from build123d import *

# Parameters (mm, degrees)
PAD_DEPTH       = 15
SKETCH001_W     = 12
SKETCH001_H     = 5.5
POCKET_DEPTH    = 12.001
SKETCH002_R     = 2.25
POCKET001_DEPTH = 20.001
CHAMFER_SIZE    = 1.5
CHAMFER001_SIZE = 2.5
CHAMFER002_SIZE = 0.5


with BuildPart() as part:
    # Sketch → Pad (new body)
    with BuildSketch(Plane.XZ):
        Polygon((-6, 20), (-4.1, 20), (-4.1, 5), (4.1, 5), (4.1, 20), (6, 20), (6, 0), (-6, 0), align=None)
    extrude(amount=PAD_DEPTH)

    # Sketch001 (on Face2 of Pad) → Pocket (cut, through all)
    with BuildSketch(Plane(origin=(6, 0, 0), x_dir=(0, 0, 1), z_dir=(1, 0, 0))):
        with Locations((13, 7.5)):
            Rectangle(SKETCH001_W, SKETCH001_H)
    extrude(amount=-POCKET_DEPTH, mode=Mode.SUBTRACT)

    # Sketch002 (on Face11 of Pocket) → Pocket001 (cut, through all)
    with BuildSketch(Plane(origin=(0, 0, 0), x_dir=(1, 0, 0), z_dir=(0, 0, -1))):
        with Locations((0, 7.5)):
            Circle(SKETCH002_R)
    extrude(amount=-POCKET001_DEPTH, mode=Mode.SUBTRACT)

    # Chamfer
    chamfer_edges = [part.edges().sort_by_distance(p)[0] for p in [
        (6, -4.75, 13),
        (6, -10.25, 13),
        (-6, -4.75, 13),
        (-6, -10.25, 13),
    ]]
    chamfer(chamfer_edges, length=CHAMFER_SIZE)

    # Chamfer001
    chamfer001_edges = [part.edges().sort_by_distance(p)[0] for p in [
        (-5.05, -15, 20),
        (5.05, -15, 20),
        (5.05, 0, 20),
        (-5.05, 0, 20),
    ]]
    chamfer(chamfer001_edges, length=CHAMFER001_SIZE)

    # Chamfer002
    chamfer002_edges = [part.edges().sort_by_distance(p)[0] for p in [
        (-2.25, -7.5, 0),
    ]]
    chamfer(chamfer002_edges, length=CHAMFER002_SIZE)


solid = part.part
Design review of the part built by this model. Coordinates are the model's own, in mm. A direction names the side the tool comes from. Coordinates: 2 decimals unless noted, no trailing zeros. Loops run counter-clockwise (first coordinate to the right, second up) from the corner with the lowest first, then second, coordinate; pieces in that order, holes last. Notation, with made-up numbers: (-37.5, 52.25) -> (17.5, 52.25) arc R12 cw to (17.5, 56.25) -> close; hole circle Ø8 at (27.25, 74.25). An arc over 180 degrees is marked (long way). Use a Markdown table: item, result. Add a question column.
Item 1: We need section B-B, the plane x = 5.25. Write out the cut boundary in (y, z).
Item 2: Wall thickness on L1, parallel to Y at x = 0, z = 2.3; L2, parallel to Z at x = -4.5, y = -9.5; L3, parallel to X at y = -2, z = 17.5: over which ranges is each line inside the solid? List them lowest first. Write a range as from..to.
Item 3: The part is to be moulded in two halves that separate along Y. For faces 1 (the flat face through (-5, -7, 19)), 2 (the flat face through (-6, -7, 5)), 3 (the flat face through (5, -1.3, 18.8)), 4 (the flat face through (5, -13.8, 18.7)), say which applies: +Y half, -Y half, draft (parallel to the pull), parting line (faces both ways), or undercut.
Item 4: Clearance check with flat-ended pins moving along their axes: P1, Ø6.5, axis at x = 0.5, y = -4.5, coming from the +Z side; P2, Ø3, axis at y = -10, z = 11, coming from the -X side; P3, Ø1, axis at x = -3, z = 16, coming from the -Y side. State where each tip first meets the part, or that it passes through.
Item 5: We need section D-D, the plane x = 0. Write out the cut boundary in (y, z).
Item 6: We need section C-C, the plane y = -1.75. Write out the cut boundary in (x, z).
Item 7: We need section A-A, the plane z = 9. Write out the cut boundary in (x, y).
Item 8: Machinability: for faces 5 (the flat face through (5.24, -4.01, 12.92)), 6 (the flat face through (-5.24, -10.99, 13.08)), 7 (the flat face through (3, -7, 0)), 8 (the flat face through (-4.1, -11, 13)), which of the approach directions +Z, -Z, +X, -X, +Y, -Y give a long, thin tool a straight path to every point of the face, cutting with its end or side? Answer none if there is none.
Numbers:
| question | item | result |
|---|---|---|
| 1 | outline | (-15, 0) -> (0, 0) -> (0, 17.5) -> (-2.5, 20) -> (-12.5, 20) -> (-15, 17.5) -> close; hole (-11, 7) -> (-4, 7) -> (-4, 19) -> (-11, 19) -> close |
| 2 | L1 | y = -15..-9.75, -5.25..0 |
| 2 | L2 | z = 0..7, 19..20 |
| 2 | L3 | x = -6..-4.1, 4.1..6 |
| 3 | face 1 | undercut |
| 3 | face 2 | draft |
| 3 | face 3 | +Y half |
| 3 | face 4 | -Y half |
| 4 | P1 | stops at z = 5 |
| 4 | P2 | stops at x = -5.75 |
| 4 | P3 | passes through |
| 5 | outline | (-15, 0) -> (-10.25, 0) -> (-9.75, 0.5) -> (-9.75, 5) -> (-15, 5) -> close; (-5.25, 0.5) -> (-4.75, 0) -> (0, 0) -> (0, 5) -> (-5.25, 5) -> close |
| 6 | outline | (-6, 0) -> (6, 0) -> (6, 19.25) -> (4.1, 19.25) -> (4.1, 5) -> (-4.1, 5) -> (-4.1, 19.25) -> (-6, 19.25) -> close |
| 7 | outline | (-6, -15) -> (-4.1, -15) -> (-4.1, -10.25) -> (-4.5, -10.25) -> (-6, -11.75) -> close; (-6, -3.25) -> (-4.5, -4.75) -> (-4.1, -4.75) -> (-4.1, 0) -> (-6, 0) -> close; (4.1, -15) -> (6, -15) -> (6, -11.75) -> (4.5, -10.25) -> (4.1, -10.25) -> close; (4.1, -4.75) -> (4.5, -4.75) -> (6, -3.25) -> (6, 0) -> (4.1, 0) -> close |
| 8 | face 5 | +X |
| 8 | face 6 | -X |
| 8 | face 7 | -Z, +X, -X, +Y, -Y |
| 8 | face 8 | +Z, +Y, -Y |
